```python
from build123d import *

# Parameters (mm, degrees)
EXTRUDE_1_DEPTH     = 8
MM_1_D              = 4
MM_1_DEPTH          = 12
MM_1_TIP            = 1.201721238
EXTRUDE_START       = -16
SKETCH_5_R          = 22.5
SKETCH_5_R_2        = 21.41
EXTRUDE_2_DEPTH     = 16
CUT_EXTRUDE_1_DEPTH = 8
CHAMFER_1_SIZE      = 8


with BuildPart() as part:
    # 草图1 → 凸台-拉伸1 (new body)
    with BuildSketch(Plane(origin=(0, 0, 0), x_dir=(0, 0, -1), z_dir=(1, 0, 0))):
        with BuildLine():
            Line((0, 0), (0, 5.59))
            ThreePointArc((0, 5.59), (-14.522523536, 11.268362763), (-21.34171621, 25.291418949))
            Line((-21.34171621, 25.291418949), (-24, 12))
            Line((-24, 12), (-24, 0))
            Line((-24, 0), (0, 0))
        make_face()
    extrude_1 = extrude(amount=-EXTRUDE_1_DEPTH)

    # 镜向1: 凸台-拉伸1 across plane
    add(extrude_1.mirror(Plane(origin=(0, 0, 0), x_dir=(1, 0, 0), z_dir=(0, 0, -1))))

    # 大小mm 暗销孔1
    with Locations(Plane(origin=(0, 0, 0), x_dir=(-1, 0, 0), z_dir=(0, -1, 0))):
        with Locations((5, 21), (5, -21)):
            Hole(MM_1_D / 2, depth=MM_1_DEPTH)
            with Locations((0, 0, -(MM_1_DEPTH + MM_1_TIP / 2))):  # 118° drill point
                Cone(0, MM_1_D / 2, MM_1_TIP, mode=Mode.SUBTRACT)

    # 草图5 → 凸台-拉伸2 (add)
    with BuildSketch(Plane.ZY.offset(8).offset(EXTRUDE_START)):
        with Locations((0, 27)):
            Circle(SKETCH_5_R)
        with Locations(Location((0, 27, 0), (0, 0, 180))):
            Circle(SKETCH_5_R_2, mode=Mode.SUBTRACT)
    extrude(amount=EXTRUDE_2_DEPTH)

    # 草图6 → 切除-拉伸1 (cut)
    with BuildSketch(Plane.ZY.offset(8)):
        Polygon((0, 27), (-12.808653102, 61.912636137), (29.307523189, 37.752264491), align=None)
    extrude(amount=-CUT_EXTRUDE_1_DEPTH, mode=Mode.SUBTRACT)

    # 倒角1
    # the kernel refuses this chamfer: 8 mm, written as the material it takes off along each edge
    with BuildSketch(Plane(origin=(-8, 41.835747499, 40.437901637), x_dir=(-0.027495876610586258, -0.938457441934671, 0.3442987168823741), z_dir=(0, -0.3444289396397119, -0.9388123910231819))) as chamfer_1_piece_1_section:
        Polygon((CHAMFER_1_SIZE * 0.999621916911, -CHAMFER_1_SIZE * 0.0274958766106), (-CHAMFER_1_SIZE * 0.0274958766106, -CHAMFER_1_SIZE * 0.999621916911), (0, 0), align=None)
    chamfer_1_piece_1 = extrude(amount=42.236927807, mode=Mode.PRIVATE)
    chamfer_1_piece_1 = split(chamfer_1_piece_1, bisect_by=Plane(origin=(0, 32.080437257, 21.522032065), z_dir=(-1, 0, 0)), keep=Keep.TOP, mode=Mode.PRIVATE)
    add(chamfer_1_piece_1, mode=Mode.SUBTRACT)
    with BuildSketch(Plane(origin=(-8, 27.785350453, -0.288127241), x_dir=(-0.02749587661058627, -0.34429871688237407, -0.9384574419346708), z_dir=(0, 0.9388123910231819, -0.34442893963971194))) as chamfer_1_piece_2_section:
        Polygon((CHAMFER_1_SIZE * 0.999621916911, -CHAMFER_1_SIZE * 0.0274958766106), (-CHAMFER_1_SIZE * 0.0274958766106, -CHAMFER_1_SIZE * 0.999621916911), (0, 0), align=None)
    chamfer_1_piece_2 = extrude(amount=42.236927807, mode=Mode.PRIVATE)
    chamfer_1_piece_2 = split(chamfer_1_piece_2, bisect_by=Plane(origin=(0, 46.701220025, -10.043437483), z_dir=(-1, 0, 0)), keep=Keep.TOP, mode=Mode.PRIVATE)
    add(chamfer_1_piece_2, mode=Mode.SUBTRACT)


solid = part.part
```
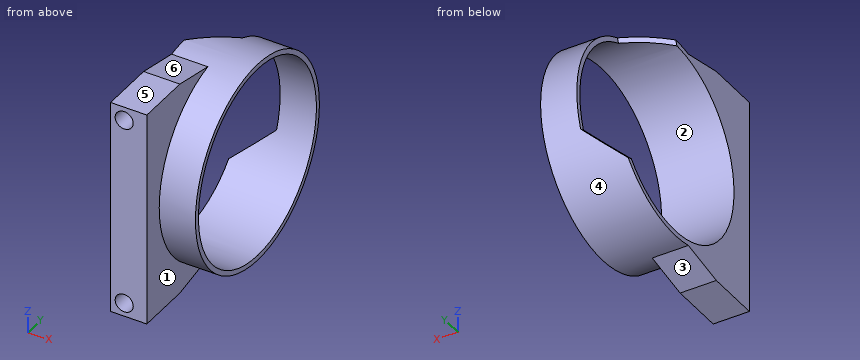
Check sheet for the modelled part. Datum: model origin and axes. Units: mm. Face numbers are marked on the shaded views. A direction names the side the tool comes from. Coordinates: 2 decimals unless noted, no trailing zeros. Order: outer loops, then holes, each group sorted by start corner. A loop starts at its lowest first (then second) coordinate and runs counter-clockwise, first axis right, second up. Notation, with made-up numbers: (-32.5, 42.5) -> (-24.5, 42.5) arc R10 cw to (-24.5, 50.5) -> close; hole circle Ø9 at (55, 80.25). An arc over 180 degrees is marked (long way). Write item = value, one per line. Start each with the question number.
1) Access from +Z, -Z, +X, -X, +Y, -Y to the whole of each face (thin tool, end or side, straight path). Record for the marked faces 4, 5 and 6.
2) Cross-section at C-C (x = -2). Enter the section's corners in (y, z).
3) Cross-section at B-B (y = 20.5). Enter the section's corners in (x, z), then the cut area to 3 significant figures.
4) Mould release check, pull along Z, two halves, no side actions. Record for the marked faces 1, 2 and 3: +Z half, -Z half, draft (parallel to the pull), parting line (faces both ways), or undercut.
5) Cross-section at A-A (z = 0). Enter the section's corners in (x, y), then the cut area to 3 significant figures.
6) Material ranges on L1, parallel to X at y = 5, z = -21; L2, parallel to Y at x = 1, z = 0; L3, parallel to Z at x = -5, y = 7.5, recorded low to high.
7) Cross-section at D-D (z = 13). Enter the section's corners in (x, y).
8) Go/stop test with flat-tipped pins: P1, Ø12, axis at y = 41, z = 4, coming from the -X side; P2, Ø2, axis at x = 4, y = 21.5, coming from the -Z side; P3, Ø5, axis at x = -4, y = 37, coming from the -Z side; P4, Ø2.5, axis at x = -5, z = 21, coming from the +Y side. Record where each tip stops, or that it passes through.
Ans:
q1.face_4 = +X
q1.face_5 = +Z, +X, -X, +Y, -Y
q1.face_6 = +Z, +X, -X
q2.outline = (0, -24) -> (12, -24) -> (22.15, -21.97) arc R22.5 ccw to (47.35, -9.6) -> (46.32, -9.22) arc R21.41 cw (long way) to (32.46, 20.7) -> (32.84, 21.73) arc R22.5 ccw to (22.15, 21.97) -> (12, 24) -> (0, 24) -> close
q3.outline = (-8, -22.3) -> (0, -22.3) -> (0, -21.54) -> (8, -21.54) -> (8, -20.4) -> (-8, -20.4) -> close; (-8, 20.4) -> (8, 20.4) -> (8, 21.54) -> (0, 21.54) -> (0, 22.3) -> (-8, 22.3) -> close
q3.area = 48.7 mm²
q4.face_1 = draft
q4.face_2 = undercut
q4.face_3 = -Z half
q5.outline = (-8, 0) -> (0, 0) -> (0, 4.5) -> (8, 4.5) -> (8, 5.59) -> (-8, 5.59) -> close; (0, 48.41) -> (8, 48.41) -> (8, 49.5) -> (0, 49.5) -> close
q5.area = 62.2 mm²
q6.L1 = -8 to -7, -3 to 0
q6.L2 = 4.5 to 5.59, 48.41 to 49.5
q6.L3 = -24 to -23, -19 to -8.84, 8.84 to 19, 23 to 24
q7.outline = (-8, 0) -> (0, 0) -> (0, 8.64) -> (8, 8.64) -> (8, 9.99) -> (-8, 9.99) -> close; (0, 44.01) -> (8, 44.01) -> (8, 45.36) -> (0, 45.36) -> close
q8.P1 = through
q8.P2 = -22.05
q8.P3 = -21.21
q8.P4 = 30.79
